```python
from build123d import *

# Parameters (mm, degrees)
PAD_DEPTH    = 2
POCKET_DEPTH = 1.5


with BuildPart() as part:
    # Sketch → Pad (new body, symmetric)
    with BuildSketch(Plane.XY):
        with BuildLine():
            ThreePointArc((21.881905, -103.28096), (26.953701, -106.209163), (29.881905, -101.137367))
            Line((29.881905, -101.137367), (5.134572, -8.779064))
            ThreePointArc((5.623337, -4.655828), (4.982691, -6.670473), (5.134572, -8.779064))
            ThreePointArc((5.623337, -4.655828), (6.272045, -0.326637), (3.986441, 3.406824))
            ThreePointArc((3.986441, 3.406824), (2.464526, 3.577404), (1.65, 2.280534))
            Line((1.65, 2.280534), (2.8, 1.616581))
            Line((2.8, -1.616581), (2.8, 1.616581))
            Line((0, -3.233162), (2.8, -1.616581))
            Line((-2.8, -1.616581), (0, -3.233162))
            Line((-2.8, 1.616581), (-2.8, -1.616581))
            Line((-1.65, 2.280534), (-2.8, 1.616581))
            ThreePointArc((-1.65, 2.280534), (-2.464526, 3.577404), (-3.986441, 3.406824))
            ThreePointArc((-3.986441, 3.406824), (-6.322816, -0.609041), (-5.327083, -5.147138))
            ThreePointArc((-3.083121, -10.110216), (-4.002626, -7.537131), (-5.327083, -5.147138))
            Line((21.881905, -103.28096), (-3.083121, -10.110216))
        make_face()
    extrude(amount=PAD_DEPTH, both=True)

    # Sketch001 → Pocket (cut)
    with BuildSketch(Plane.XY.offset(2)):
        with BuildLine():
            Line((-1.297143, -9.820912), (23.620571, -102.815086))
            ThreePointArc((23.620571, -102.815086), (26.487827, -104.470497), (28.143238, -101.603241))
            Line((28.143238, -101.603241), (3.348593, -9.068367))
            ThreePointArc((3.348593, -9.068367), (0.649453, -7.121772), (-1.297143, -9.820912))
        make_face()
    pocket = extrude(amount=-POCKET_DEPTH, mode=Mode.SUBTRACT)

    # Mirrored: Pocket across XY
    add(pocket.mirror(Plane.XY), mode=Mode.SUBTRACT)


solid = part.part
```
Could you check a few things on this model? Use its own coordinates, in mm. A direction names the side the tool comes from. Round coordinates to 2 decimals unless told otherwise and drop trailing zeros. Loops run counter-clockwise (first coordinate to the right, second up) from the corner with the lowest first, then second, coordinate; pieces in that order, holes last. Notation, with made-up numbers: (-9.5, 6.5) - (8.5, 6.5) arc R11 cw to (8.5, 18.5) - close; hole circle Ø10 at (-32.5, 19). An arc over 180 degrees is marked (long way). Answer as CSV lines item,"result".
1. Please list where these lines run through material, in increasing order: line 1 along X through (y, z) = (-57.5, -1.75); line 2 along X through (y, z) = (-73, 1.8); line 3 along Z through (x, y) = (10, -35.5). Write a range as [from, to].
Filled in:
line 1,"x = [9.61, 11.48], [16.33, 18.19]"
line 2,"x = [13.77, 15.63], [20.48, 22.34]"
line 3,"z = [-0.5, 0.5]"
2. We'd pull the mould along Y, two halves only. Please class faces 5 (the face through (13, -43, -2)), 6 (the face through (-3.99, -7.57, 0.03)), 7 (the face through (-2.444, 3.567, 0.028)), 8 (the face through (13, -56, 0.5)): +Y half, -Y half, draft (parallel to the pull), parting line (faces both ways), or undercut.
Filled in:
face 5,"draft"
face 6,"-Y half"
face 7,"+Y half"
face 8,"undercut"
3. I want a section at B-B on x = 19. List the corners of the cut face in (y, z) for me.
Filled in:
outline,"(-92.53, -2) - (-85.57, -2) - (-85.57, -0.5) - (-67.48, -0.5) - (-67.48, -2) - (-60.53, -2) - (-60.53, 2) - (-67.48, 2) - (-67.48, 0.5) - (-85.57, 0.5) - (-85.57, 2) - (-92.53, 2) - close"
4. For pin 1 Ø1.6 at (y, z) = (0, -0.5) entering from +X; pin 2 Ø2 at (y, z) = (-56, 0) entering from +X; pin 3 Ø1 at (y, z) = (-58, 1.5) entering from -X; pin 4 Ø5 at (x, y) = (20.5, -52.5) entering from -Z, each with a flat end and sliding along its axis, tell me the tip position at first contact or that it passes through.
Filled in:
pin 1,"stops at x = 6.35"
pin 2,"stops at x = 18.06"
pin 3,"stops at x = 9.61"
pin 4,"passes through"
5. I want a section at A-A on y = -25. List the corners of the cut face in (x, z) for me.
Filled in:
outline,"(0.91, -2) - (2.77, -2) - (2.77, -0.5) - (7.62, -0.5) - (7.62, -2) - (9.48, -2) - (9.48, 2) - (7.62, 2) - (7.62, 0.5) - (2.77, 0.5) - (2.77, 2) - (0.91, 2) - close"
6. On a 3-axis mill with a long thin cutter (end or side, diameter ignored), from which of +Z, -Z, +X, -X, +Y, -Y can I reach the whole of each face in a straight line? I mean faces 1 (the face through (2.485, 3.587, 0.028)), 2 (the face through (1.38, -2.436, 0.028)), 3 (the face through (15.92, -55.98, 1.26)), 4 (the face through (15.92, -55.98, -1.26)). Say none if no direction works.
Filled in:
face 1,"+Z, -Z, +Y"
face 2,"+Z, -Z"
face 3,"+Z"
face 4,"-Z"
